Input: part model. Units: mm. Frame: model coordinates. Round coordinates to 2 decimals unless told otherwise and drop trailing zeros. Loops run counter-clockwise (first coordinate to the right, second up) from the corner with the lowest first, then second, coordinate; pieces in that order, holes last. Notation, with made-up numbers: M 4.5,33 L 8.5,33 A14 ccw 8.5,49 Z; hole C 25,-15 d10. An arc over 180 degrees is marked long. Use one line per item in the form item = value. Start each with the question number.
Q1. First-contact query: P1, Ø5, axis at x = 65, y = 0, coming from the +Z side; P2, Ø0.9, axis at y = 50.5, z = 2, coming from the +X side; P3, Ø1.5, axis at x = -34.5, z = 1, coming from the -Y side; P4, Ø2.5, axis at x = 0, y = 65, coming from the +Z side. Flat tips, straight axial feed; report the tip coordinate or a pass-through.
Q2. Section query A-A, the plane z = 1.05. Output: boundary loops of the cut face in (x, y).
Q3. Ray query, line 1 along Y through (x, z) = (0, 1.9); line 2 along Y through (x, z) = (65, 1.2); line 3 along X through (y, z) = (36, 0.75). Return the intervals inside material, ascending.
Q4. Section query C-C, the plane x = -39.5. Output: boundary loops of the cut face in (y, z).
Q5. Section query B-B, the plane y = 36.5. Output: boundary loops of the cut face in (x, z), and give its area (3 significant figures).
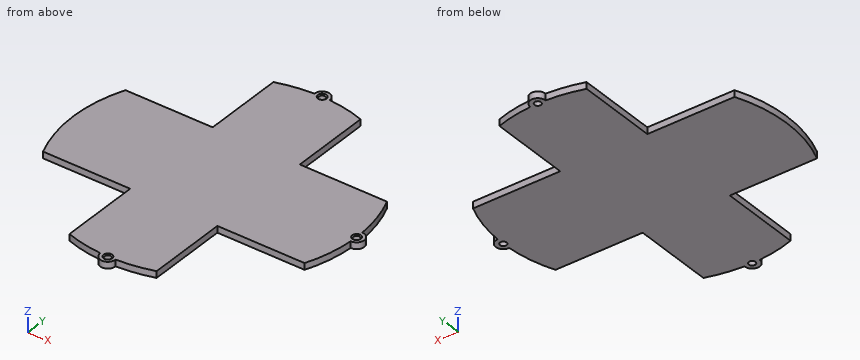
```python
from build123d import *

# Parameters (mm, degrees)
EXTRUDE_1_DEPTH     = 3
SKETCH_2_R          = 3.5
EXTRUDE_2_DEPTH     = 3
SKETCH_3_R          = 1.5
CUT_EXTRUDE_1_DEPTH = 3
CHAMFER_1_SIZE      = 0.5


with BuildPart() as part:
    # 草图1 → 凸台-拉伸1 (new body)
    with BuildSketch(Plane.XY):
        with BuildLine():
            Line((20, -25), (20, -61.846584384))
            ThreePointArc((20, -61.846584384), (0, -65), (-20, -61.846584384))
            Line((-20, -61.846584384), (-20, -25))
            Line((-20, -25), (-60, -25))
            ThreePointArc((-60, -25), (-65, 0), (-60, 25))
            Line((-60, 25), (-20, 25))
            Line((-20, 25), (-20, 61.846584384))
            ThreePointArc((-20, 61.846584384), (0, 65), (20, 61.846584384))
            Line((20, 61.846584384), (20, 25))
            Line((20, 25), (60, 25))
            ThreePointArc((60, 25), (65, 0), (60, -25))
            Line((60, -25), (20, -25))
        make_face()
    extrude(amount=EXTRUDE_1_DEPTH)

    # 草图2 → 凸台-拉伸2 (add)
    with BuildSketch(Plane.XY.offset(3)):
        with Locations((65, 0)):
            Circle(SKETCH_2_R)
        with Locations((0, 65)):
            Circle(SKETCH_2_R)
        with Locations((0, -65)):
            Circle(SKETCH_2_R)
    extrude(amount=-EXTRUDE_2_DEPTH)

    # 草图3 → 切除-拉伸1 (cut)
    with BuildSketch(Plane.XY.offset(3)):
        with Locations((0, 65)):
            Circle(SKETCH_3_R)
        with Locations((65, 0)):
            Circle(SKETCH_3_R)
        with Locations((0, -65)):
            Circle(SKETCH_3_R)
    extrude(amount=-CUT_EXTRUDE_1_DEPTH, mode=Mode.SUBTRACT)

    # 倒角1
    chamfer_1_edges = [part.edges().sort_by_distance(p)[0] for p in [
        (-1.5, 65, 3),
        (63.5, 0, 3),
        (-1.5, -65, 3),
    ]]
    chamfer(chamfer_1_edges, length=CHAMFER_1_SIZE)


solid = part.part
```
Results found:
q1.P1 = 3
q1.P2 = 20
q1.P3 = -25
q1.P4 = through
q2.outline = M -60,-25 L -20,-25 L -20,-61.85 A65 ccw -3.5,-64.91 A3.5 ccw long 3.5,-64.91 A65 ccw 20,-61.85 L 20,-25 L 60,-25 A65 ccw 64.91,-3.5 A3.5 ccw long 64.91,3.5 A65 ccw 60,25 L 20,25 L 20,61.85 A65 ccw 3.5,64.91 A3.5 ccw long -3.5,64.91 A65 ccw -20,61.85 L -20,25 L -60,25 A65 ccw Z; hole C 0,-65 d3; hole C 0,65 d3; hole C 65,0 d3
q3.line_1 = -68.5 to -66.5, -63.5 to 63.5, 66.5 to 68.5
q3.line_2 = -3.5 to -1.5, 1.5 to 3.5
q3.line_3 = -20 to 20
q4.outline = M -25,0 L 25,0 L 25,3 L -25,3 Z
q5.outline = M -20,0 L 20,0 L 20,3 L -20,3 Z
q5.area = 120 mm²
